Verification items for the finished model (mm, model axes). Face numbers are marked on the shaded views. Round coordinates to 2 decimals unless told otherwise and drop trailing zeros. Write each loop counter-clockwise with the first axis right and the second up, starting at its lowest first coordinate (ties: lowest second). Pieces come first, ordered by that corner, then holes. Notation, with made-up numbers: M -17.5,87.5 L 21.5,87.5 A23 cw 21.5,123.5 Z; hole C 35.25,82 d3. An arc over 180 degrees is marked long. Write each question's results on one line, items separated by ' | '.
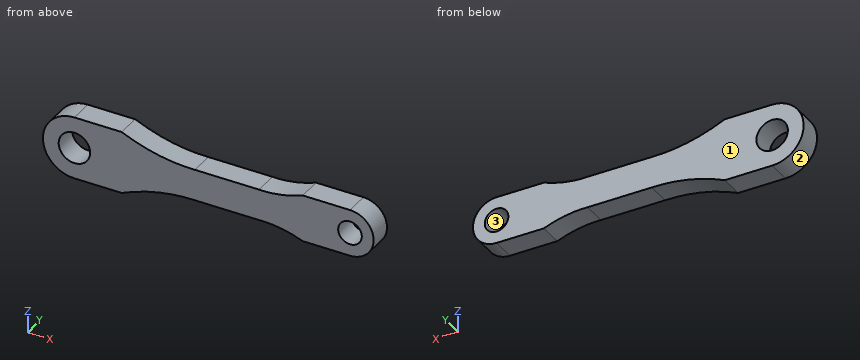
from build123d import *

# Parameters (mm, degrees)
SKETCH1_R           = 2
SKETCH1_R_2         = 1.5
BOSS_EXTRUDE1_DEPTH = 3


with BuildPart() as part:
    # Sketch1 → Boss-Extrude1 (new body)
    with BuildSketch(Plane(origin=(0, 0, 0), x_dir=(1, 0, 0), z_dir=(0, 1, 0))):
        with BuildLine():
            Line((-17.5, -4), (-11.5, -4))
            add(Edge.make_bspline(
                [(-11.5, -4), (-8.431864047, -2.610600203), (-5.332163957, -1.943933537), (-2.200899734, -2)],
                knots=[0, 0, 0, 0, 0.616300928, 0.616300928, 0.616300928, 0.616300928], degree=3))
            Line((-2.200899734, -2), (5.947351403, -2))
            add(Edge.make_bspline(
                [(11.5, -3), (9.673149322, -2.269768842), (7.822266456, -1.936435509), (5.947351403, -2)],
                knots=[0, 0, 0, 0, 0.698718256, 0.698718256, 0.698718256, 0.698718256], degree=3))
            Line((11.5, -3), (17.5, -3))
            ThreePointArc((17.5, -3), (20.5, 0), (17.5, 3))
            Line((17.5, 3), (11.5, 3))
            add(Edge.make_bspline(
                [(11.5, 3), (9.673149322, 2.269768842), (7.822266456, 1.936435509), (5.947351403, 2)],
                knots=[0, 0, 0, 0, 0.698718256, 0.698718256, 0.698718256, 0.698718256], degree=3))
            Line((5.947351403, 2), (-2.200899734, 2))
            add(Edge.make_bspline(
                [(-11.5, 4), (-8.431864047, 2.610600203), (-5.332163957, 1.943933537), (-2.200899734, 2)],
                knots=[0, 0, 0, 0, 0.616300928, 0.616300928, 0.616300928, 0.616300928], degree=3))
            Line((-11.5, 4), (-17.5, 4))
            ThreePointArc((-17.5, 4), (-21.5, 0), (-17.5, -4))
        make_face()
        with Locations(Location((-17.5, 0, 0), (0, 0, 270))):
            Circle(SKETCH1_R, mode=Mode.SUBTRACT)
        with Locations(Location((17.5, 0, 0), (0, 0, 270))):
            Circle(SKETCH1_R_2, mode=Mode.SUBTRACT)
    extrude(amount=BOSS_EXTRUDE1_DEPTH)


solid = part.part
1) Sectioned sample at A-A, the plane z = 0. Record the cut outline in (x, y).
Calculated:
outline: M -21.5,0 L -19.5,0 L -19.5,3 L -21.5,3 Z; M -15.5,0 L 16,0 L 16,3 L -15.5,3 Z; M 19,0 L 20.5,0 L 20.5,3 L 19,3 Z
2) Depth check by flat-ended pin: P1, Ø1.5, axis at x = 2, y = 2, coming from the +Z side; P2, Ø1.5, axis at y = 0.5, z = 3, coming from the -X side; P3, Ø1.5, axis at y = 2.5, z = 1, coming from the -X side; P4, Ø2.5, axis at x = -17.5, z = 0, coming from the -Y side. Enter the tip coordinate at first touch or a pass-through.
Calculated:
P1: stops at z = 2 | P2: stops at x = -20.81 | P3: stops at x = -21.49 | P4: passes through
3) Draft check along Z on the marked faces 1, 2 and 3. Enter one of: pulls with the +Z half, pulls with the -Z half, needs draft (parallel to the pull), parting line crosses it, or undercut.
Calculated:
face 1: needs draft | face 2: parting line crosses it | face 3: undercut
4) Sectioned sample at D-D, the plane y = 1.75. Count the separate pieces of the cut face and the enclosed holes in it, and give its area (3 significant figures).
Calculated:
separate pieces: 1 | enclosed holes: 2 | area: 211 mm²
5) Sectioned sample at B-B, the plane x = -16. Record the cut outline in (y, z).
Calculated:
outline: M 0,-4 L 3,-4 L 3,-1.32 L 0,-1.32 Z; M 0,1.32 L 3,1.32 L 3,4 L 0,4 Z
6) Sectioned sample at C-C, the plane x = 15. Record the cut outline in (y, z).
Calculated:
outline: M 0,-3 L 3,-3 L 3,3 L 0,3 Z
7) Material ranges on line 1 (X direction, y = 0.9, z = 0); line 2 (X direction, y = 2.4, z = -0.5); line 3 (Z direction, x = 14.5, y = 0.5), recorded low to high. Write a range as [from, to].
Calculated:
line 1: x = [-21.5, -19.5], [-15.5, 16], [19, 20.5] | line 2: x = [-21.47, -19.44], [-15.56, 16.09], [18.91, 20.46] | line 3: z = [-3, 3]
